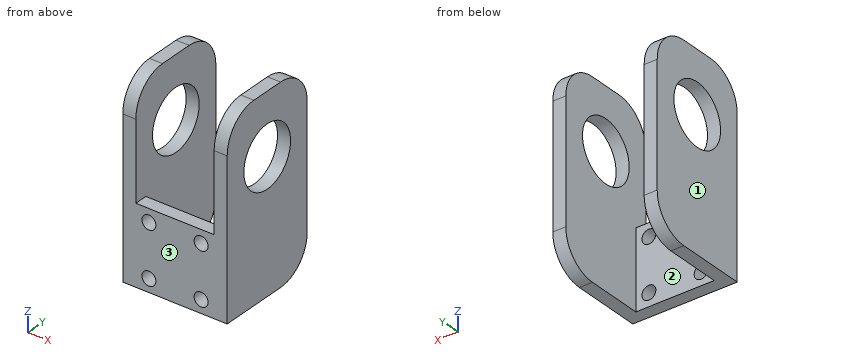
Autodesk Inventor part; units mm, degrees
ref_plane "YZ Plane" through (0, 0, 0) normal (1, 0, 0) x (0, 1, 0)
ref_plane "XZ Plane" through (0, 0, 0) normal (0, 1, 0) x (-1, 0, 0)
ref_plane "XY Plane" through (0, 0, 0) normal (0, 0, 1) x (1, 0, 0)
sketch "Sketch1" plane through (0, 0, 0) normal (0, 0, 1) x (1, 0, 0)
  line L0 (-19.05, 38.1) -> (-14.2875, 38.1)
  line L1 (-14.2875, 38.1) -> (-14.2875, 4.7625)
  line L2 (-14.2875, 4.7625) -> (14.2875, 4.7625)
  line L3 (14.2875, 4.7625) -> (14.2875, 38.1)
  line L4 (14.2875, 38.1) -> (19.05, 38.1)
  line L5 (19.05, 38.1) -> (19.05, 0)
  line L6 (19.05, 0) -> (-19.05, 0)
  line L7 (-19.05, 0) -> (-19.05, 38.1)
  line L8 (0, 0) -> (0, 4.7625) construction
  dimension "d0" = 4.7625
  dimension "d2" = 38.1
  dimension "d3" = 38.1
extrude "Extrusion1" add sketch "Sketch1" along normal blind 69.85
sketch "Sketch2" plane through (-14.2875, 4.7625, 0) normal (0, 1, 0) x (1, 0, 0)
  line L0 (23.8125, -23.8125) -> (4.7625, -23.8125) construction
  line L1 (4.7625, -23.8125) -> (4.7625, -4.7625) construction
  line L2 (4.7625, -4.7625) -> (23.8125, -4.7625) construction
  line L3 (23.8125, -4.7625) -> (23.8125, -23.8125) construction
  line L4 (23.8125, -23.8125) -> (4.7625, -4.7625) construction
  line L5 (4.7625, -23.8125) -> (23.8125, -4.7625) construction
  circle A0 centre (4.7625, -4.7625) radius 2.54
  circle A1 centre (4.7625, -23.8125) radius 2.54
  circle A2 centre (23.8125, -4.7625) radius 2.54
  circle A3 centre (23.8125, -23.8125) radius 2.54
  line L6 (0, 0) -> (0, -69.85)
  line L7 (28.575, 0) -> (28.575, -69.85)
  line L8 (0, -69.85) -> (28.575, -69.85)
  line L9 (28.575, -69.85) -> (28.575, -28.575)
  line L10 (28.575, -28.575) -> (0, -28.575)
  line L11 (0, -28.575) -> (0, -69.85)
  line L12 (14.2875, -4.7625) -> (14.2875, 0) construction
  point P0 (14.2875, -14.2875)
  dimension "d6" = 5.08
  dimension "d7" = 19.05
  dimension "d8" = 19.05
  dimension "d10" = 14.2875
  dimension "d21" = 4.7625
  dimension "d22" = 4.7625
extrude "Extrusion2" cut sketch "Sketch2" against normal through all
sketch "Sketch3" plane through (19.05, 0, 0) normal (1, 0, 0) x (0, 0, -1)
  circle A0 centre (-47.625, 19.05) radius 11.1125
  circle A1 centre (-47.625, 19.05) radius 14.2875 construction
  line L0 (-33.3375, 19.05) -> (-33.3375, -6.9181) construction
  line L1 (0, 0) -> (-69.85, 0) construction
  dimension "d15" = 28.575
  dimension "d13" = 22.225
  dimension "d14" = 19.05
  dimension "d16" = 33.3375
extrude "Extrusion3" cut sketch "Sketch3" against normal through all
fillet "Fillet1" radius 12.7 6 edges at (16.6687, 38.1, 69.85) (-16.6687, 38.1, 69.85) (16.6687, 38.1, 0) (-16.6687, 38.1, 0) (-16.6688, 0, 69.85) (16.6688, 0, 69.85)
properties part number "top pully bracket" material "Aluminum 6061"
Build history of the part. All positions in model axes, mm. Face numbers are marked on the shaded views. Round coordinates to 2 decimals unless told otherwise and drop trailing zeros. Write each loop counter-clockwise with the first axis right and the second up, starting at its lowest first coordinate (ties: lowest second). Pieces come first, ordered by that corner, then holes. Notation, with made-up numbers: (-16.75, 3) - (-0.75, 3) arc R32 cw to (-0.75, 31) - close; hole circle Ø2 at (-15, 58). An arc over 180 degrees is marked (long way). Write each question's results on one line, items separated by ' | '. Start each with the question number.
Item 1: Wall check: L1, parallel to X at y = 13, z = 31.5; L2, parallel to Y at x = -17, z = 38.5; L3, parallel to Z at x = -17, y = 19. Give the ranges that are in metal, low to high. Write a range as [from, to].
Item 2: Saw through at A-A (y = 19.05). Write the cut outline in (x, z).
Item 3: Mould opens along X. For the marked faces 1, 2 and 3 say: pulls with the +X half, pulls with the -X half, needs draft (parallel to the pull), parting line crosses it, or undercut.
Item 4: Saw through at C-C (z = 6). Write the cut outline in (x, y), and give its area (3 significant figures).
Item 5: Saw through at B-B (x = 9). Write the cut outline in (y, z) (1 decimal), and give its area (3 significant figures).
Item 6: Drop flat-ended pins along their axis: P1, Ø1, axis at x = 12.5, y = 5.5, coming from the -Z side; P2, Ø1, axis at x = 5.5, z = 10.5, coming from the +Y side; P3, Ø5, axis at x = -5, y = 1.5, coming from the +Z side (3 decimals). Give the stop position or say it passes through.
Item 7: Saw through at D-D (z = 48.5). Write the cut outline in (x, y).
Results are:
1) L1: x = [-19.05, -14.29], [14.29, 19.05] | L2: y = [0, 12.71], [25.39, 38.1] | L3: z = [0, 36.51], [58.74, 69.85]
2) outline: (-19.05, 0) - (-14.29, 0) - (-14.29, 36.51) - (-19.05, 36.51) - close; (-19.05, 58.74) - (-14.29, 58.74) - (-14.29, 69.85) - (-19.05, 69.85) - close; (14.29, 0) - (19.05, 0) - (19.05, 36.51) - (14.29, 36.51) - close; (14.29, 58.74) - (19.05, 58.74) - (19.05, 69.85) - (14.29, 69.85) - close
3) face 1: pulls with the -X half | face 2: undercut | face 3: needs draft
4) outline: (-19.05, 0) - (-11.74, 0) - (-11.74, 4.76) - (-14.29, 4.76) - (-14.29, 36.19) - (-19.05, 36.19) - close; (-7.31, 0) - (7.31, 0) - (7.31, 4.76) - (-7.31, 4.76) - close; (11.74, 0) - (19.05, 0) - (19.05, 36.19) - (14.29, 36.19) - (14.29, 4.76) - (11.74, 4.76) - close | area: 439 mm²
5) outline: (0, 0) - (4.8, 0) - (4.8, 2.3) - (0, 2.3) - close; (0, 7.2) - (4.8, 7.2) - (4.8, 21.3) - (0, 21.3) - close; (0, 26.3) - (4.8, 26.3) - (4.8, 28.6) - (0, 28.6) - close | area: 88.7 mm²
6) P1: passes through | P2: stops at y = 4.76 | P3: stops at z = 28.575
7) outline: (-19.05, 0) - (-14.29, 0) - (-14.29, 7.97) - (-19.05, 7.97) - close; (-19.05, 30.13) - (-14.29, 30.13) - (-14.29, 38.1) - (-19.05, 38.1) - close; (14.29, 0) - (19.05, 0) - (19.05, 7.97) - (14.29, 7.97) - close; (14.29, 30.13) - (19.05, 30.13) - (19.05, 38.1) - (14.29, 38.1) - close
